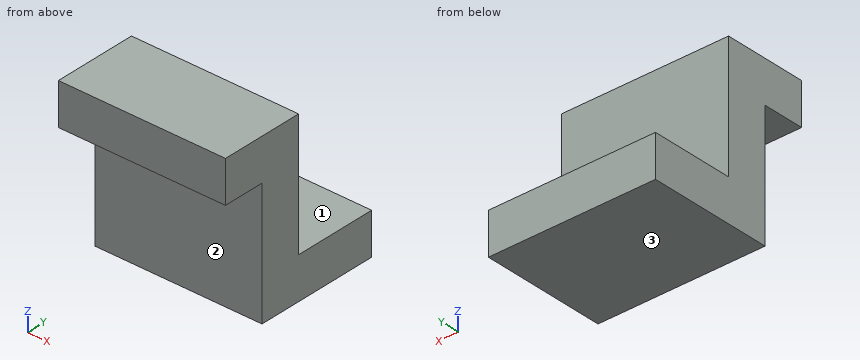
from build123d import *

# Parameters (mm, degrees)
F0_W     = 101.6
F0_H     = 101.6
F1_DEPTH = 76.2
F3_W     = 101.6
F3_H     = 25.4
F4_DEPTH = 25.4
F2_W     = 50.8
F2_H     = 76.2
F5_DEPTH = 101.6


with BuildPart() as f1:
    # F0 (on Front) → F1 (new body)
    with BuildSketch(Plane.XZ):
        with Locations((-50.8, 50.8)):
            Rectangle(F0_W, F0_H)
    extrude(amount=F1_DEPTH)

    # F3 (on face) → F4 (join)
    with BuildSketch(Plane.XZ.offset(76.2)):
        with Locations((-50.8, 88.9)):
            Rectangle(F3_W, F3_H)
    extrude(amount=F4_DEPTH)

    # F2 (on face) → F5 (cut)
    with BuildSketch(Plane.YZ):
        with Locations((-25.4, 63.5)):
            Rectangle(F2_W, F2_H)
    extrude(amount=-F5_DEPTH, mode=Mode.SUBTRACT)


solid = f1.part
Could you check a few things on this model? Use its own coordinates, in mm. Face numbers are marked on the shaded views. A direction names the side the tool comes from. Round coordinates to 2 decimals unless told otherwise and drop trailing zeros. Write each loop counter-clockwise with the first axis right and the second up, starting at its lowest first coordinate (ties: lowest second). Pieces come first, ordered by that corner, then holes. Notation, with made-up numbers: (58.25, 76) -> (74.25, 76) arc R22 ccw to (74.25, 107) -> close; hole circle Ø11 at (20, -1). An arc over 180 degrees is marked (long way). Use a Markdown table: item, result.
1. For pin 1 Ø23 at (x, z) = (-43.5, 59.5) entering from +Y; pin 2 Ø12.5 at (x, y) = (-38, -87.5) entering from -Z, each with a flat end and sliding along its axis, tell me the tip position at first contact or that it passes through.
Answer key:
| item | result |
|---|---|
| pin 1 | stops at y = -50.8 |
| pin 2 | stops at z = 76.2 |
2. Please list where these lines run through material, in increasing order: probe 1 along Y at (x, z) = (-78.5, 92.5); probe 2 along Y at (x, z) = (-67, 30); probe 3 along Z at (x, y) = (-84, -36.5).
Answer key:
| item | result |
|---|---|
| probe 1 | y = -101.6 to -50.8 |
| probe 2 | y = -76.2 to -50.8 |
| probe 3 | z = 0 to 25.4 |
3. If we section it at B-B (z = 56): List the corners of the cut face in (x, y) for me, then the cut area to 3 significant figures.
Answer key:
| item | result |
|---|---|
| outline | (-101.6, -76.2) -> (0, -76.2) -> (0, -50.8) -> (-101.6, -50.8) -> close |
| area | 2,580 mm^2 |
4. Which directions (+Z, -Z, +X, -X, +Y, -Y) give clear straight access to the entire face, cutting with the end or side of a thin tool? Please do the marked faces 1, 2 and 3.
Answer key:
| item | result |
|---|---|
| face 1 | +Z, +X, -X, +Y |
| face 2 | -Z, +X, -X, -Y |
| face 3 | -Z, +X, -X, +Y, -Y |
5. If we section it at A-A (x = -7): List the corners of the cut face in (y, z) for me, then the cut area to 3 significant figures.
Answer key:
| item | result |
|---|---|
| outline | (-101.6, 76.2) -> (-76.2, 76.2) -> (-76.2, 0) -> (0, 0) -> (0, 25.4) -> (-50.8, 25.4) -> (-50.8, 101.6) -> (-101.6, 101.6) -> close |
| area | 4,520 mm^2 |
6. If we section it at C-C (y = -11): List the corners of the cut face in (x, z) for me, then the cut area to 3 significant figures.
Answer key:
| item | result |
|---|---|
| outline | (-101.6, 0) -> (0, 0) -> (0, 25.4) -> (-101.6, 25.4) -> close |
| area | 2,580 mm^2 |
